Could you check a few things on this model? Use its own coordinates, in mm. A direction names the side the tool comes from. Give positions to 0.01 mm unless a question says otherwise; leave off trailing zeros. Write each loop counter-clockwise with the first axis right and the second up, starting at its lowest first coordinate (ties: lowest second). Pieces come first, ordered by that corner, then holes. Notation, with made-up numbers: (-36.5, 82) - (8.5, 82) arc R11 cw to (8.5, 94) - close; hole circle Ø6 at (29.5, 48). An arc over 180 degrees is marked (long way). Write item = value, one per line.
from build123d import *

# Parameters (mm, degrees)
SKETCH2_W            = 66.35
SKETCH2_H            = 66
BOSS_EXTRUDE1_DEPTH  = 3.175
CUT_EXTRUDE1_DEPTH   = 47.900546372
M3_CLEARANCE_HOLE1_D = 3.2
SKETCH7_W            = 3.225
SKETCH7_H            = 8.1
CUT_EXTRUDE2_DEPTH   = 47.900546372
SKETCH8_W            = 8
SKETCH8_H            = 3.175
BOSS_EXTRUDE2_DEPTH  = 3.175
FILLET1_R            = 1
FILLET2_R            = 1


with BuildPart() as part:
    # Sketch2 → Boss-Extrude1 (new body)
    with BuildSketch(Plane(origin=(0, 0, 0), x_dir=(0, 0, -1), z_dir=(1, 0, 0))):
        Rectangle(SKETCH2_W, SKETCH2_H)
    extrude(amount=BOSS_EXTRUDE1_DEPTH)

    # Sketch3 → Cut-Extrude1 (cut, through all)
    with BuildSketch(Plane(origin=(3.175, 0, 0), x_dir=(0, 0, -1), z_dir=(1, 0, 0))):
        Polygon((-20, -20), (-20, -33), (20, -33), (20, -20), (20, 20), (-20, 20), align=None)
    extrude(amount=-CUT_EXTRUDE1_DEPTH, mode=Mode.SUBTRACT)

    # M3 Clearance Hole1 (through all)
    with Locations(Plane(origin=(3.175, 0, 0), x_dir=(0, 0, -1), z_dir=(1, 0, 0))):
        with Locations((-25, -29.5), (25, -29.5)):
            Hole(M3_CLEARANCE_HOLE1_D / 2)

    # Sketch7 → Cut-Extrude2 (cut, through all)
    with BuildSketch(Plane(origin=(3.175, 0, 0), x_dir=(0, 0, -1), z_dir=(1, 0, 0))):
        with Locations((-31.5625, 15)):
            Rectangle(SKETCH7_W, SKETCH7_H)
        with Locations((-31.5625, -15)):
            Rectangle(SKETCH7_W, SKETCH7_H)
        with Locations((31.5625, -15)):
            Rectangle(SKETCH7_W, SKETCH7_H)
        with Locations((31.5625, 15)):
            Rectangle(SKETCH7_W, SKETCH7_H)
    extrude(amount=-CUT_EXTRUDE2_DEPTH, mode=Mode.SUBTRACT)

    # Sketch8 → Boss-Extrude2 (add)
    with BuildSketch(Plane(origin=(3.175, 0, 0), x_dir=(0, 0, -1), z_dir=(1, 0, 0))):
        with Locations((-15, 34.5875)):
            Rectangle(SKETCH8_W, SKETCH8_H)
        with Locations((15, 34.5875)):
            Rectangle(SKETCH8_W, SKETCH8_H)
    extrude(amount=-BOSS_EXTRUDE2_DEPTH)

    # Fillet1
    fillet1_edges = [part.edges().sort_by_distance(p)[0] for p in [
        (1.5875, 20, -20),
        (1.5875, 20, 20),
    ]]
    fillet(fillet1_edges, radius=FILLET1_R)

    # Fillet2
    fillet2_edges = [part.edges().sort_by_distance(p)[0] for p in [
        (1.5875, -33, -20),
        (1.5875, -33, 20),
        (1.5875, -33, -33.175),
        (1.5875, -33, 33.175),
        (1.5875, 33, 33.175),
        (1.5875, 33, -33.175),
    ]]
    fillet(fillet2_edges, radius=FILLET2_R)


solid = part.part
1. I need wall thicknesses on line 1 (Z direction, x = 1.2, y = -23.5) (3 decimals); line 2 (Z direction, x = 2.7, y = -19); line 3 (Y direction, x = 1, z = -25). Which ranges of each line are inside material? Lowest first, please.
Filled sheet:
line_1 = -33.175 to -20, 20 to 33.175
line_2 = -29.95 to -20, 20 to 29.95
line_3 = -33 to -31.1, -27.9 to 33
2. If we section it at A-A, the plane y = -29.5: Please give me the cut outline in (x, z) (3 decimals), and give its area (3 significant figures).
Filled sheet:
outline = (0, -33.175) - (3.175, -33.175) - (3.175, -26.6) - (0, -26.6) - close; (0, -23.4) - (3.175, -23.4) - (3.175, -20) - (0, -20) - close; (0, 20) - (3.175, 20) - (3.175, 23.4) - (0, 23.4) - close; (0, 26.6) - (3.175, 26.6) - (3.175, 33.175) - (0, 33.175) - close
area = 63.3 mm2
3. If we section it at C-C, the plane y = -6: Please give me the cut outline in (x, z) (3 decimals).
Filled sheet:
outline = (0, -33.175) - (3.175, -33.175) - (3.175, -20) - (0, -20) - close; (0, 20) - (3.175, 20) - (3.175, 33.175) - (0, 33.175) - close
4. Which directions (+Z, -Z, +X, -X, +Y, -Y) give clear straight access to the entire face, cutting with the end or side of a thin tool? Please do faces 5 (the face through (2, 10.95, 32)), 6 (the face through (2, 15, -29.95)), 7 (the face through (2, 20, 0)).
Filled sheet:
face_5 = +Z, +X, -X
face_6 = -Z, +X, -X
face_7 = +X, -X, -Y
5. If we section it at D-D, the plane z = -9: Please give me the cut outline in (x, y) (3 decimals).
Filled sheet:
outline = (0, 20) - (3.175, 20) - (3.175, 33) - (0, 33) - close
6. Thinking about a two-plate mould opening in Y: for faces 1 (the face through (2, -33, 27)), 2 (the face through (2, -19.05, -32)), 3 (the face through (2, 25, 33.175)), 4 (the face through (2, 36.175, -15)), which applies, pulls with the +Y half, pulls with the -Y half, needs draft (parallel to the pull), parting line crosses it, or undercut?
Filled sheet:
face_1 = pulls with the -Y half
face_2 = undercut
face_3 = needs draft
face_4 = pulls with the +Y half
7. If we section it at B-B, the plane z = -25: Please give me the cut outline in (x, y) (3 decimals).
Filled sheet:
outline = (0, -33) - (3.175, -33) - (3.175, -31.1) - (0, -31.1) - close; (0, -27.9) - (3.175, -27.9) - (3.175, 33) - (0, 33) - close
8. For pin 1 (1 mm diameter, centred on x = 1, z = 32, fed in from +Y); pin 2 (1.6 mm diameter, centred on x = 1, y = 34.5, fed in from -Z); pin 3 (1 mm diameter, centred on x = 1.5, y = -15, fed in from +Z), each with a flat end and sliding along its axis, tell me the tip position at first contact or that it passes through.
Filled sheet:
pin_1 = 33
pin_2 = -19
pin_3 = 29.95
